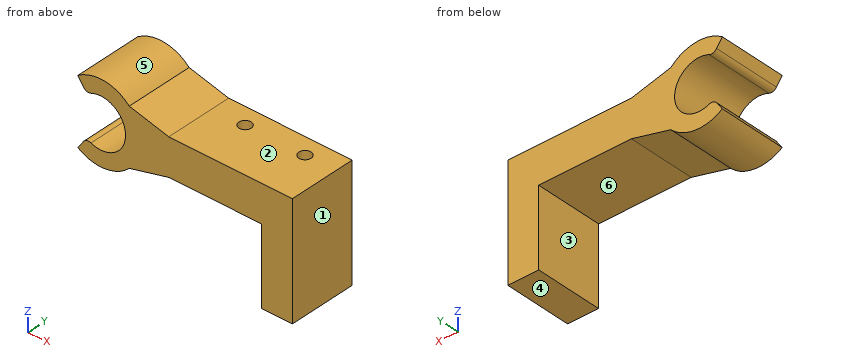
```python
from build123d import *

# Parameters (mm, degrees)
ESQUISSE1_W             = 20
ESQUISSE1_H             = 6
BOSS_EXTRU_1_DEPTH      = 11
ESQUISSE2_R             = 1
ENL_V_MAT_EXTRU_1_DEPTH = 4
ESQUISSE3_W             = 5
ESQUISSE3_H             = 11
BOSS_EXTRU_2_DEPTH      = 12.5


with BuildPart() as part:
    # Esquisse1 → Boss.-Extru.1 (new body)
    with BuildSketch(Plane(origin=(0, 0, 0), x_dir=(1, 0, 0), z_dir=(0, 1, 0))):
        with Locations((21, 0)):
            Rectangle(ESQUISSE1_W, ESQUISSE1_H)
        with BuildLine():
            Line((11, -3), (11, 3))
            Line((11, 3), (4.596194078, 4.596194078))
            ThreePointArc((4.596194078, 4.596194078), (0.566512328, 6.475265538), (-3.728246836, 5.324488288))
            Line((-3.728246836, 5.324488288), (-2.809939195, 4.013009061))
            ThreePointArc((-2.809939195, 4.013009061), (-2.262538006, 3.624217858), (-1.592629721, 3.669268398))
            ThreePointArc((-1.592629721, 3.669268398), (4, 0), (-1.592629721, -3.669268398))
            ThreePointArc((-1.592629721, -3.669268398), (-2.262538006, -3.624217858), (-2.809939195, -4.013009061))
            Line((-2.809939195, -4.013009061), (-3.728246836, -5.324488288))
            ThreePointArc((-3.728246836, -5.324488288), (0.566512328, -6.475265538), (4.596194078, -4.596194078))
            Line((4.596194078, -4.596194078), (11, -3))
        make_face()
    extrude(amount=BOSS_EXTRU_1_DEPTH)

    # Esquisse2 → Enlèv. mat.-Extru.1 (cut)
    with BuildSketch(Plane.XY.offset(3)):
        with Locations((16.3, 8)):
            Circle(ESQUISSE2_R)
        with Locations((26, 8)):
            Circle(ESQUISSE2_R)
    extrude(amount=-ENL_V_MAT_EXTRU_1_DEPTH, mode=Mode.SUBTRACT)

    # Esquisse3 → Boss.-Extru.2 (add)
    with BuildSketch(Plane(origin=(0, 0, -3), x_dir=(-1, 0, 0), z_dir=(0, 0, -1))):
        with Locations((-28.5, 5.5)):
            Rectangle(ESQUISSE3_W, ESQUISSE3_H)
    extrude(amount=BOSS_EXTRU_2_DEPTH)


solid = part.part
```
The listing builds one solid part. Answer for the finished solid, in the listing's coordinates (mm). Face numbers are marked on the shaded views. A direction names the side the tool comes from. Give positions to 0.01 mm unless a question says otherwise; leave off trailing zeros. Loops run counter-clockwise (first coordinate to the right, second up) from the corner with the lowest first, then second, coordinate; pieces in that order, holes last. Notation, with made-up numbers: (59, -32.5) - (106, -32.5) arc R12 cw to (106, -20.5) - close; hole circle Ø9 at (-18, 13). An arc over 180 degrees is marked (long way). Return JSON: item names as keys, results as strings. Group by question number.
1. Which of the six approach directions +Z, -Z, +X, -X, +Y, -Y give full straight-line access (tool end or side, diameter ignored) to the marked faces 1, 2 and 3?
2. Find section B-B (z = 0). Write down the section's boundary in (x, y), then the cut area to 3 significant figures.
3. Find section A-A (x = 0). Write down the section's boundary in (y, z), then the cut area to 3 significant figures.
4. Given pin 1 Ø1.5 at (x, y) = (6, 9) entering from -Z; pin 2 Ø0.6 at (x, y) = (26, 7.5) entering from +Z; pin 3 Ø5.5 at (x, y) = (15.5, 8) entering from -Z, each flat-ended and moving along its own axis, determine where each tip first touches the part or whether it passes through.
5. Find section C-C (x = 16.3). Write down the section's boundary in (y, z), then the cut area to 3 significant figures.
6. Find section D-D (y = 6.5). Write down the section's boundary in (x, z), then the cut area to 3 significant figures.
7. Straight lines are drawn through the part: line 1 (Z direction, x = 0, y = 3.5); line 2 (Y direction, x = 16.3, z = 0.8); line 3 (Z direction, x = 29, y = 8.5). For each, find the intervals that lie inside material, in ascending order. Write a range as [from, to].
8. Determine the mould class of the marked faces 4, 5 and 6 for opening direction X: pulls with the +X half, pulls with the -X half, needs draft (parallel to the pull), parting line crosses it, or undercut.
Verdict:
{
 "1": {"face 1": "+Z, -Z, +X, +Y, -Y", "face 2": "+Z, +X, +Y, -Y", "face 3": "-Z, +Y, -Y"},
 "2": {"outline": "(4, 0) - (31, 0) - (31, 11) - (4, 11) - close; hole circle Ø2 at (16.3, 8); hole circle Ø2 at (26, 8)", "area": "291 mm^2"},
 "3": {"outline": "(0, -6.5) - (11, -6.5) - (11, -4) - (0, -4) - close; (0, 4) - (11, 4) - (11, 6.5) - (0, 6.5) - close", "area": "55.0 mm^2"},
 "4": {"pin 1": "stops at z = -4.43", "pin 2": "stops at z = -1", "pin 3": "stops at z = -3"},
 "5": {"outline": "(0, -3) - (11, -3) - (11, 3) - (9, 3) - (9, -1) - (7, -1) - (7, 3) - (0, 3) - close", "area": "58.0 mm^2"},
 "6": {"outline": "(-3.73, -5.32) arc R6.5 ccw to (4.6, -4.6) - (11, -3) - (26, -3) - (26, -15.5) - (31, -15.5) - (31, 3) - (11, 3) - (4.6, 4.6) arc R6.5 ccw to (-3.73, 5.32) - (-2.81, 4.01) arc R1 ccw to (-1.59, 3.67) arc R4 cw (long way) to (-1.59, -3.67) arc R1 ccw to (-2.81, -4.01) - close", "area": "276 mm^2"},
 "7": {"line 1": "z = [-6.5, -4], [4, 6.5]", "line 2": "y = [0, 7], [9, 11]", "line 3": "z = [-15.5, 3]"},
 "8": {"face 4": "needs draft", "face 5": "parting line crosses it", "face 6": "undercut"}
}
